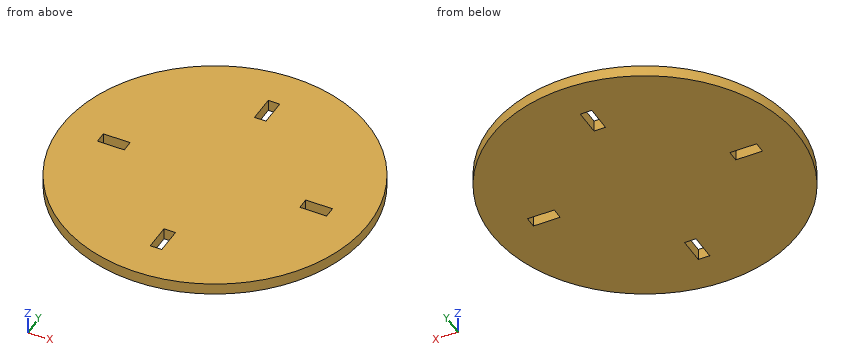
from build123d import *

# Parameters (mm, degrees)
F0_R     = 508
F1_DEPTH = 38.1
F2_W     = 88.9
F2_H     = 38.1
F2_W_2   = 38.1
F2_H_2   = 88.9
F3_DEPTH = 38.101


with BuildPart() as f1:
    # F0 (on Top) → F1 (new body)
    with BuildSketch(Plane.XY):
        Circle(F0_R)
    extrude(amount=-F1_DEPTH)

    # F2 (on face) → F3 (cut, through all)
    with BuildSketch(Plane(origin=(0, 0, -38.1), x_dir=(1, 0, 0), z_dir=(0, 0, -1))):
        with Locations((-336.073452, 0)):
            Rectangle(F2_W, F2_H)
        with Locations((0, -336.073452)):
            Rectangle(F2_W_2, F2_H_2)
        with Locations((336.073452, 0)):
            Rectangle(F2_W, F2_H)
        with Locations((0, 336.073452)):
            Rectangle(F2_W_2, F2_H_2)
    extrude(amount=-F3_DEPTH, mode=Mode.SUBTRACT)


solid = f1.part
Check sheet for the modelled part. Datum: model origin and axes. Units: mm. Round coordinates to 2 decimals unless told otherwise and drop trailing zeros. Loops run counter-clockwise (first coordinate to the right, second up) from the corner with the lowest first, then second, coordinate; pieces in that order, holes last.
1. Sectioned sample at A-A on x = 0. Record the boundary of the cut face in (y, z).
2. Sectioned sample at D-D on x = 144. Record the boundary of the cut face in (y, z).
3. Gauge pin test, flat ends, axial feed: pin 1 Ø1 at (x, z) = (-331, -6.5) entering from +Y; pin 2 Ø5 at (y, z) = (-267.5, -18) entering from +X; pin 3 Ø19 at (x, z) = (-358, -18) entering from +Y. Record the tip position at first contact, or that the pin passes through.
4. Sectioned sample at C-C on z = -8. Record the boundary of the cut face in (x, y).
5. Scan lines: probe 1 along X at (y, z) = (11, -8); probe 2 along Y at (x, z) = (17, -30.5); probe 3 along X at (y, z) = (-332, -9). Record each from-to range of solid material in increasing order.
Recorded:
1. outline: (-508, -38.1) - (-380.52, -38.1) - (-380.52, 0) - (-508, 0) - close; (-291.62, -38.1) - (291.62, -38.1) - (291.62, 0) - (-291.62, 0) - close; (380.52, -38.1) - (508, -38.1) - (508, 0) - (380.52, 0) - close
2. outline: (-487.16, -38.1) - (487.16, -38.1) - (487.16, 0) - (-487.16, 0) - close
3. pin 1: stops at y = 385.79
3. pin 2: stops at x = 433.4
3. pin 3: stops at y = 369.61
4. outline: circle Ø1016 at (0, 0); hole (-380.52, -19.05) - (-291.62, -19.05) - (-291.62, 19.05) - (-380.52, 19.05) - close; hole (-19.05, -380.52) - (19.05, -380.52) - (19.05, -291.62) - (-19.05, -291.62) - close; hole (-19.05, 291.62) - (19.05, 291.62) - (19.05, 380.52) - (-19.05, 380.52) - close; hole (291.62, -19.05) - (380.52, -19.05) - (380.52, 19.05) - (291.62, 19.05) - close
5. probe 1: x = -507.88 to -380.52, -291.62 to 291.62, 380.52 to 507.88
5. probe 2: y = -507.72 to -380.52, -291.62 to 291.62, 380.52 to 507.72
5. probe 3: x = -384.5 to -19.05, 19.05 to 384.5
